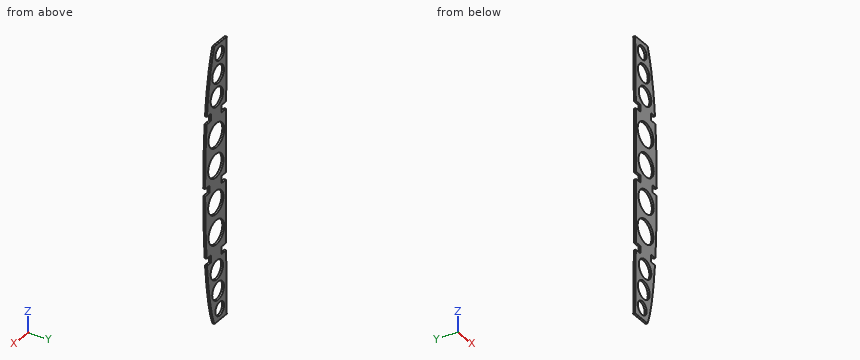
from build123d import *

# Parameters (mm, degrees)
F0_R     = 19.603688
F0_R_2   = 13.870468
F0_R_3   = 18.530739
F0_R_4   = 24.78659
F0_R_5   = 24.059578
F1_DEPTH = 4


with BuildPart() as f1:
    # F0 (on Front) → F1 (new body)
    with BuildSketch(Plane.XZ):
        with BuildLine():
            Line((247.598545, 129.316792), (218.598545, 129.316792))
            Line((218.598545, 129.316792), (208.598545, 129.316792))
            add(Edge.make_bspline(
                [(208.598545, 129.316792), (209.292892, 85.650126), (209.987238, 41.983459), (210.532804, -1.683208)],
                knots=[0, 0, 0, 0, 131.00736, 131.00736, 131.00736, 131.00736], degree=3))
            Line((210.532804, -1.683208), (224.714136, -1.683208))
            Line((224.714136, -1.683208), (224.714136, -9.183208))
            Line((224.714136, -9.183208), (258.207463, -9.183208))
            Line((258.207463, -9.183208), (258.207463, -1.683208))
            Line((258.207463, -1.683208), (271.015688, -1.683208))
            add(Edge.make_bspline(
                [(247.598545, 129.316792), (258.936994, 97.14756), (266.473841, 51.345555), (271.015688, -1.683208)],
                knots=[0, 0, 0, 0, 151.505652, 151.505652, 151.505652, 151.505652], degree=3))
        make_face()
        with Locations((239.830866, 22.773052)):
            Circle(F0_R, mode=Mode.SUBTRACT)
        with Locations((230.733871, 106.829256)):
            Circle(F0_R_2, mode=Mode.SUBTRACT)
        with Locations((235.828176, 67.530252)):
            Circle(F0_R_3, mode=Mode.SUBTRACT)
        with BuildLine():
            Line((258.207463, -16.683208), (258.207463, -9.183208))
            Line((258.207463, -9.183208), (224.714136, -9.183208))
            Line((224.714136, -9.183208), (224.714136, -16.683208))
            Line((224.714136, -16.683208), (210.714136, -16.683208))
            add(Edge.make_bspline(
                [(210.714136, -16.683208), (211.217845, -59.849874), (211.559513, -103.016541), (211.595413, -146.183208)],
                knots=[146.008203, 146.008203, 146.008203, 146.008203, 275.515479, 275.515479, 275.515479, 275.515479], degree=3))
            Line((211.595413, -146.183208), (225.595413, -146.183208))
            Line((225.595413, -146.183208), (225.595413, -153.683208))
            Line((225.595413, -153.683208), (262.598491, -153.683208))
            Line((262.598491, -153.683208), (262.598491, -146.183208))
            Line((262.598491, -146.183208), (276.598491, -146.183208))
            add(Edge.make_bspline(
                [(272.207463, -16.683208), (275.174253, -57.063181), (276.527478, -101.107051), (276.598491, -146.183208)],
                knots=[165.616704, 165.616704, 165.616704, 165.616704, 278.243078, 278.243078, 278.243078, 278.243078], degree=3))
            Line((272.207463, -16.683208), (258.207463, -16.683208))
        make_face()
        with Locations((241.286382, -54.733325)):
            Circle(F0_R_4, mode=Mode.SUBTRACT)
        with Locations((243.105769, -116.228998)):
            Circle(F0_R_5, mode=Mode.SUBTRACT)
        with BuildLine():
            add(Edge.make_bspline(
                [(210.532804, -305.683208), (209.987238, -349.349874), (209.292892, -393.016541), (208.598545, -436.683208)],
                knots=[435.024441, 435.024441, 435.024441, 435.024441, 566.031801, 566.031801, 566.031801, 566.031801], degree=3))
            Line((208.598545, -436.683208), (218.598545, -436.683208))
            Line((218.598545, -436.683208), (247.598545, -436.683208))
            add(Edge.make_bspline(
                [(270.954375, -305.683208), (266.376933, -362.117906), (258.822956, -409.911712), (247.598545, -436.683208)],
                knots=[413.826682, 413.826682, 413.826682, 413.826682, 568.963971, 568.963971, 568.963971, 568.963971], degree=3))
            Line((270.954375, -305.683208), (258.207463, -305.683208))
            Line((258.207463, -305.683208), (258.207463, -298.183208))
            Line((258.207463, -298.183208), (258.207463, -290.683208))
            Line((258.207463, -290.683208), (272.08775, -290.683208))
            add(Edge.make_bspline(
                [(276.575303, -161.183208), (276.370496, -205.212088), (274.956086, -249.83193), (272.08775, -290.683208)],
                knots=[290.707653, 290.707653, 290.707653, 290.707653, 400.255998, 400.255998, 400.255998, 400.255998], degree=3))
            Line((276.575303, -161.183208), (262.598491, -161.183208))
            Line((262.598491, -161.183208), (262.598491, -153.683208))
            Line((262.598491, -153.683208), (225.595413, -153.683208))
            Line((225.595413, -153.683208), (225.595413, -161.183208))
            Line((225.595413, -161.183208), (211.595413, -161.183208))
            add(Edge.make_bspline(
                [(211.595413, -161.183208), (211.559513, -204.349874), (211.217845, -247.516541), (210.714136, -290.683208)],
                knots=[290.516322, 290.516322, 290.516322, 290.516322, 420.023598, 420.023598, 420.023598, 420.023598], degree=3))
            Line((210.714136, -290.683208), (224.714136, -290.683208))
            Line((224.714136, -290.683208), (224.714136, -305.683208))
            Line((224.714136, -305.683208), (210.532804, -305.683208))
        make_face()
        with Locations((230.733871, -414.195671)):
            Circle(F0_R_2, mode=Mode.SUBTRACT)
        with Locations((235.828176, -374.896667)):
            Circle(F0_R_3, mode=Mode.SUBTRACT)
        with Locations((239.830866, -330.139467)):
            Circle(F0_R, mode=Mode.SUBTRACT)
        with Locations((241.286382, -252.633091)):
            Circle(F0_R_4, mode=Mode.SUBTRACT)
        with Locations((243.105769, -191.137418)):
            Circle(F0_R_5, mode=Mode.SUBTRACT)
    extrude(amount=F1_DEPTH)


solid = f1.part
Work out the finished part from the listing and answer in its coordinate system (mm). Round coordinates to 2 decimals unless told otherwise and drop trailing zeros. Use one line per item in the form item = value.
(1) Find section A-A on y = -2.4. Give the number of separate pieces and of enclosed holes in the cut face, then the cut area to 3 significant figures.
Answer list:
separate_pieces = 1
enclosed_holes = 10
area = 18,600 mm2
(2) Straight lines are drawn through the part: line 1 (Z direction, x = 215, y = -1.15); line 2 (X direction, y = -2.5, z = -56.5); line 3 (X direction, y = -2.45, z = -114). For each, find the intervals that lie inside material, in ascending order.
Answer list:
line_1 = -436.68 to -305.68, -290.68 to -161.18, -146.18 to -16.68, -1.68 to 129.32
line_2 = 211.13 to 216.56, 266.01 to 274.57
line_3 = 211.51 to 219.15, 267.06 to 276.32
(3) Flat-ended cylindrical pins translate along their axes: P1, Ø2, axis at y = -1.5, z = -153.5, coming from the -X side; P2, Ø2, axis at y = -1.5, z = -298.5, coming from the +X side. Find the tip coordinate at first contact, or state that the pin passes through.
Answer list:
P1 = 225.6
P2 = 258.21
